Part model, mm, in its own coordinate system. A direction names the side the tool comes from. Coordinates: 2 decimals unless noted, no trailing zeros. Loops run counter-clockwise (first coordinate to the right, second up) from the corner with the lowest first, then second, coordinate; pieces in that order, holes last. Notation, with made-up numbers: (44, -2.75) -> (71, -2.75) arc R27 ccw to (71, 20.25) -> close; hole circle Ø3 at (29.25, 4.5). An arc over 180 degrees is marked (long way). Use one line per item in the form item = value. Start each with the question number.
(1) Drill centre lines: L1, parallel to Y at x = 0, z = 35; L2, parallel to Y at x = 0, z = 34.5; L3, parallel to X at y = 17, z = 51. Where is each one in solid material? Low to high. Write a range as [from, to].
(2) 3-axis set-ups, long thin cutter, end or side, ignore diameter. For faces 1 (the cylindrical face through (23.9, -7.5, 37)), 2 (the flat face through (0, 0, 75)): which of +Z, -Z, +X, -X, +Y, -Y reach the whole face in a straight line?
(3) Mould opens along Y. For faces 3 (the flat face through (6.54, -24.34, 75)), 4 (the cylindrical face through (-16.989, -15.578, 36.975)), 5 (the conical face through (-36.1, -8, 62)) say: +Y half, -Y half, draft (parallel to the pull), parting line (faces both ways), or undercut.
(4) Band-saw the part on A-A on y = 0. Give the cut face in (x, z), then the cut area to 3 significant figures.
(5) Pin check, flat tips, straight feed: P1, Ø1.5, axis at x = -29.5, z = 63.5, coming from the +Y side; P2, Ø1, axis at y = -23, z = 15, coming from the +X side; P3, Ø4, axis at x = 50, y = 41, coming from the +Z side. Stop position of each tip, or through.
(6) Band-saw the part on B-B on z = 57.5. Give the cut face in (x, y), then the cut area to 3 significant figures.
(7) Band-saw the part on D-D on z = 30.5. Give the cut face in (x, y), then the cut area to 3 significant figures.
Autodesk Inventor part; units mm, degrees
ref_plane "YZ Plane" through (0, 0, 0) normal (1, 0, 0) x (0, 1, 0)
ref_plane "XZ Plane" through (0, 0, 0) normal (0, 1, 0) x (-1, 0, 0)
ref_plane "XY Plane" through (0, 0, 0) normal (0, 0, 1) x (1, 0, 0)
sketch "Skizze1" plane through (0, 0, 0) normal (0, 0, 1) x (1, 0, 0)
  circle A0 centre (0, 0) radius 70
  circle A1 centre (0, 0) radius 25.05
  circle A2 centre (0, 0) radius 23.05
  dimension "d0" = 140
  dimension "d1" = 50.1
  dimension "d2" = 46.1
extrude "Extrusion1" add sketch "Skizze1" against normal blind 5 contours A0 | A1 | A2
extrude "Extrusion2" add sketch "Skizze1" along normal blind 75
sketch "Skizze2" plane through (0, 0, 0) normal (1, 0, 0) x (0, 1, 0)
  line L0 (23.05, 75) -> (23.05, 0)
  line L1 (23.05, 0) -> (25.05, 0)
  line L2 (25.05, 0) -> (25.05, 75)
  line L3 (25.05, 75) -> (70, 75)
  line L4 (70, 75) -> (70, -5)
  line L5 (70, -5) -> (-70, -5)
  line L6 (-70, -5) -> (-70, 75)
  line L7 (-70, 75) -> (-25.05, 75)
  line L8 (-25.05, 75) -> (-25.05, 0)
  line L9 (-25.05, 0) -> (-23.05, 0)
  line L10 (-23.05, 0) -> (-23.05, 75)
  line L11 (-23.05, 75) -> (23.05, 75)
  line L12 (70, 75) -> (70, 0)
  line L13 (0, 75) -> (0, -5) construction
  line L14 (70, 0) -> (30.05, 75)
  line L15 (70, 75) -> (30.05, 75)
  point P0 (0, 0)
  dimension "d7" = 5
revolve "Umdrehung1" cut sketch "Skizze2" angle 360 about axis through (0, 0, 75) along (0, 0, -1) contours L3 L4 L14
properties part number "Zyklon_Konus"
A:
q1.L1 = [-51.36, -25.05], [-23.05, 23.05], [25.05, 51.36]
q1.L2 = [-51.62, -25.05], [-23.05, 23.05], [25.05, 51.62]
q1.L3 = [-39.32, -18.4], [-15.57, 15.57], [18.4, 39.32]
q2.face_1 = +Z
q2.face_2 = +Z, +X, -X, +Y, -Y
q3.face_3 = draft
q3.face_4 = undercut
q3.face_5 = parting line
q4.outline = (-70, -5) -> (70, -5) -> (70, 0) -> (30.05, 75) -> (25.05, 75) -> (25.05, 0) -> (23.05, 0) -> (23.05, 75) -> (-23.05, 75) -> (-23.05, 0) -> (-25.05, 0) -> (-25.05, 75) -> (-30.05, 75) -> (-70, 0) -> close
q4.area = 7,900 mm²
q5.P1 = 22.16
q5.P2 = 57.93
q5.P3 = 13.78
q6.outline = circle Ø78.74 at (0, 0); circle Ø46.1 at (0, 0); hole circle Ø50.1 at (0, 0)
q6.area = 4,570 mm²
q7.outline = circle Ø107.51 at (0, 0); circle Ø46.1 at (0, 0); hole circle Ø50.1 at (0, 0)
q7.area = 8,780 mm²
